Answer from the drawing. Dimensions are ordinates in mm from the lowest x, y and z of the part. A direction names the side the tool comes from. Give positions to 0.01 mm unless a question says otherwise; leave off trailing zeros. Write each loop counter-clockwise with the first axis right and the second up, starting at its lowest first coordinate (ties: lowest second). Pieces come first, ordered by that corner, then holes.
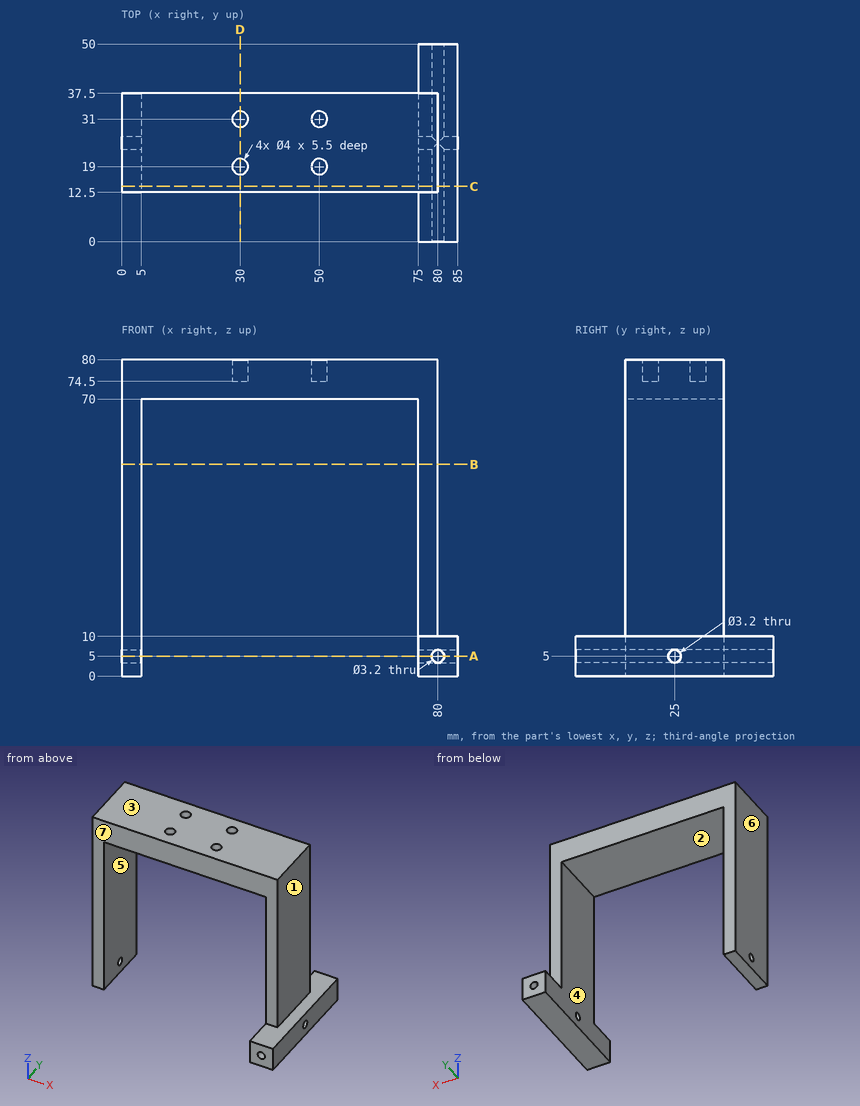
Item 1: Section C-C (y = 14) is taken. Write down the section's boundary in (x, z), and give its area (3 significant figures).
Result set:
outline: (0, 0) - (5, 0) - (5, 70) - (75, 70) - (75, 0) - (85, 0) - (85, 10) - (80, 10) - (80, 80) - (0, 80) - close; hole circle Ø3.2 at (80, 5)
area: 1,540 mm2
Item 2: Section A-A (z = 5) is taken. Write down the section's boundary in (x, y), and give its area (3 significant figures).
Result set:
outline: (0, 12.5) - (5, 12.5) - (5, 23.4) - (0, 23.4) - close; (0, 26.6) - (5, 26.6) - (5, 37.5) - (0, 37.5) - close; (75, 0) - (78.4, 0) - (78.4, 23.4) - (75, 23.4) - close; (75, 26.6) - (78.4, 26.6) - (78.4, 50) - (75, 50) - close; (81.6, 0) - (85, 0) - (85, 23.4) - (81.6, 23.4) - close; (81.6, 26.6) - (85, 26.6) - (85, 50) - (81.6, 50) - close
area: 427 mm2
Item 3: Section D-D (x = 30) is taken. Write down the section's boundary in (y, z).
Result set:
outline: (12.5, 70) - (37.5, 70) - (37.5, 80) - (33, 80) - (33, 74.5) - (29, 74.5) - (29, 80) - (21, 80) - (21, 74.5) - (17, 74.5) - (17, 80) - (12.5, 80) - close
Item 4: Section B-B (z = 53.5) is taken. Write down the section's boundary in (x, y).
Result set:
outline: (0, 12.5) - (5, 12.5) - (5, 37.5) - (0, 37.5) - close; (75, 12.5) - (80, 12.5) - (80, 37.5) - (75, 37.5) - close
Item 5: Which of the six approach directions +Z, -Z, +X, -X, +Y, -Y give full straight-line access (tool end or side, diameter ignored) to the marked faces 1, 2 and 3?
Result set:
face 1: +Z, +X, +Y, -Y
face 2: -Z, +Y, -Y
face 3: +Z, +X, -X, +Y, -Y
Item 6: Find the intervals of material crossed by line 1 along Y through (x, z) = (50, 78.6); line 2 along X through (y, z) = (19, 78.45); line 3 along X through (y, z) = (37, 13), in increasing order.
Result set:
line 1: y = 12.5 to 17, 21 to 29, 33 to 37.5
line 2: x = 0 to 28, 32 to 48, 52 to 80
line 3: x = 0 to 5, 75 to 80
Item 7: Determine the mould class of the marked faces 4, 5, 6 and 7 for opening direction X: pulls with the +X half, pulls with the -X half, needs draft (parallel to the pull), parting line crosses it, or undercut.
Result set:
face 4: undercut
face 5: undercut
face 6: pulls with the -X half
face 7: needs draft
Item 8: Each of these flat-tipped pins is pushed along its axis until it touches: pin 1 Ø6 at (y, z) = (33, 47.5) entering from +X; pin 2 Ø1.5 at (y, z) = (24, 55.5) entering from -X; pin 3 Ø5 at (x, y) = (30, 31) entering from -Z; pin 4 Ø3.5 at (x, y) = (50, 31) entering from +Z. Where does it stop, or does it pass through?
Result set:
pin 1: stops at x = 80
pin 2: stops at x = 0
pin 3: stops at z = 70
pin 4: stops at z = 74.5
